from build123d import *

# Parameters (mm, degrees)
BOSS_EXTRUDE1_DEPTH = 12
SKETCH2_W           = 130
SKETCH2_H           = 30
SKETCH2_W_2         = 170
SKETCH2_H_2         = 15
CUT_EXTRUDE1_DEPTH  = 609.394608786
CHAMFER1_SIZE       = 12


with BuildPart() as part:
    # Sketch1 → Boss-Extrude1 (new body)
    with BuildSketch(Plane.XY):
        with BuildLine():
            Line((0, 0), (0, -10))
            Line((0, -10), (40, -10))
            ThreePointArc((40, -10), (48.819660113, -2.639320225), (60, 0))
            Line((60, 0), (540, 0))
            ThreePointArc((540, 0), (551.180339887, -2.639320225), (560, -10))
            Line((560, -10), (600, -10))
            Line((600, -10), (600, 0))
            Line((600, 0), (600, 100))
            Line((600, 100), (0, 100))
            Line((0, 100), (0, 0))
        make_face()
    extrude(amount=BOSS_EXTRUDE1_DEPTH)

    # Sketch2 → Cut-Extrude1 (cut, through all)
    with BuildSketch(Plane.XY.offset(12)):
        with Locations((110, 50)):
            Rectangle(SKETCH2_W, SKETCH2_H)
        with Locations((300, 50)):
            Rectangle(SKETCH2_W_2, SKETCH2_H_2)
        with Locations((490, 50)):
            Rectangle(SKETCH2_W, SKETCH2_H)
    extrude(amount=-CUT_EXTRUDE1_DEPTH, mode=Mode.SUBTRACT)

    # Chamfer1
    chamfer1_edges = [part.edges().sort_by_distance(p)[0] for p in [
        (600, 45, 12),
        (300, 100, 12),
        (0, 45, 12),
    ]]
    chamfer(chamfer1_edges, length=CHAMFER1_SIZE - 0.0001)  # a hair under: the kernel refuses the full size


solid = part.part
The model under review builds one solid part; all positions refer to its coordinate system, in mm. A direction names the side the tool comes from. Round coordinates to 2 decimals unless told otherwise and drop trailing zeros. Order: outer loops, then holes, each group sorted by start corner. A loop starts at its lowest first (then second) coordinate and runs counter-clockwise, first axis right, second up. Notation, with made-up numbers: (45.5, 24) -> (83.5, 24) arc R13 cw to (83.5, 28) -> close; hole circle Ø5 at (-14.75, 7). An arc over 180 degrees is marked (long way). Use CSV: the item, a comma, the result in double quotes. Start each with the question number.
(1) Mouldability with a two-part tool opening along Y and no side actions: class faces 1 (the face through (24, -10, 6)), 2 (the face through (385, 50, 6)), 3 (the face through (109, 65, 6)), 4 (the face through (296, 40, 12)) as pulls with the +Y half, pulls with the -Y half, needs draft (parallel to the pull), parting line crosses it, or undercut.
(2) Wall thickness on probe 1 along X at (y, z) = (40, 11.75); probe 2 along X at (y, z) = (60, 1.75); probe 3 along Y at (x, z) = (236, 3): over which ranges is each line inside the solid? List them lowest first. Write a range as from..to.
(3) Consider section B-B on z = 5.25. Write out the cut boundary in (x, y), and give its area (3 significant figures).
(4) Tool access review of faces 5 (the face through (551.035, -2.567, 5.916)), 6 (the face through (296, 58, 0)), 7 (the face through (175, 50, 6)): name each direction out of +Z, -Z, +X, -X, +Y, -Y from which nothing blocks a thin tool from reaching the whole face with its end or side.
(5) Insertion check: pin 1 (6 mm diameter, centred on y = 3, z = 2.5, fed in from +X); pin 2 (3.5 mm diameter, centred on x = 283.5, z = 7.5, fed in from -Y); pin 3 (6 mm diameter, centred on y = 49, z = 3.5, fed in from -X). Each pin has a flat end and moves straight along its axis. Give the tip position at first contact, or say it passes through.
Responses:
1,face 1,"pulls with the -Y half"
1,face 2,"undercut"
1,face 3,"undercut"
1,face 4,"needs draft"
2,probe 1,"11.75..45, 175..425, 555..588.25"
2,probe 2,"1.75..45, 175..425, 555..598.25"
2,probe 3,"0..42.5, 57.5..97"
3,outline,"(5.25, -10) -> (40, -10) arc R25 cw to (60, 0) -> (540, 0) arc R25 cw to (560, -10) -> (594.75, -10) -> (594.75, 94.75) -> (5.25, 94.75) -> close; hole (45, 35) -> (175, 35) -> (175, 65) -> (45, 65) -> close; hole (215, 42.5) -> (385, 42.5) -> (385, 57.5) -> (215, 57.5) -> close; hole (425, 35) -> (555, 35) -> (555, 65) -> (425, 65) -> close"
3,area,"46,300 mm²"
4,face 5,"+Z, -Z, -Y"
4,face 6,"-Z, +X, -X, +Y, -Y"
4,face 7,"+Z, -Z"
5,pin 1,"x = 600"
5,pin 2,"y = 0"
5,pin 3,"x = 0.5"
